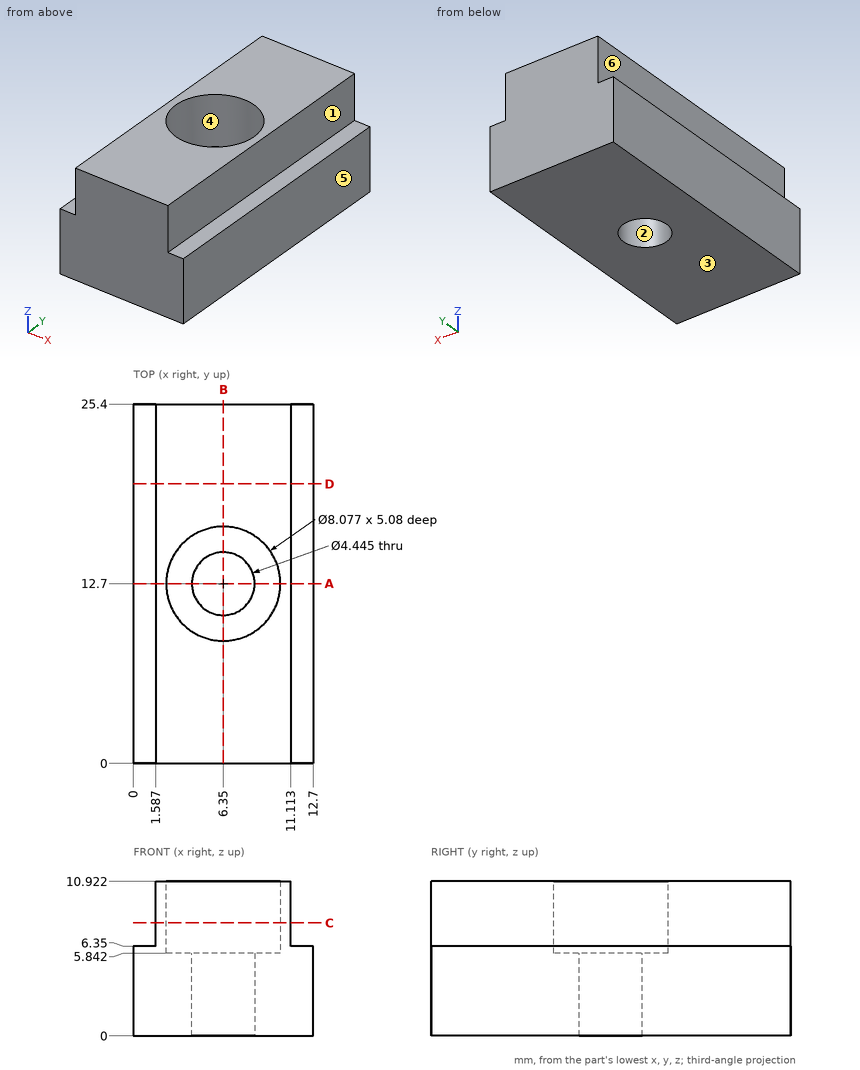
Here's the drawing with two shaded views (mm, measured from the low corner). I have some questions. A direction names the side the tool comes from. Give positions to 0.01 mm unless a question says otherwise; leave off trailing zeros. Order: outer loops, then holes, each group sorted by start corner. A loop starts at its lowest first (then second) coordinate and runs counter-clockwise, first axis right, second up.
Q1. I'm going to push flat-ended pins straight in: P1, Ø2.5, axis at x = 6.35, y = 12.7, coming from the -Z side; P2, Ø5, axis at x = 6.35, y = 12.7, coming from the +Z side; P3, Ø1.4, axis at y = 13.5, z = 9, coming from the -X side. Where does each tip first touch, or does it pass through?
Q2. If I drill on line 1 along Y through (x, z) = (6.35, 9.45); line 2 along Y through (x, z) = (6.35, 2.4); line 3 along Z through (x, y) = (5.5, 10.5), over which ranges is the centre line in solid material (lowest first)?
Q3. Suppose I cut it at A-A, the plane y = 12.7. Write out the boundary of the cut face in (x, z).
Q4. Suppose I cut it at C-C, the plane z = 8. Write out the boundary of the cut face in (x, y), and give its area (3 significant figures).
Q5. We'd pull the mould along X, two halves only. Please class the marked faces 3, 4, 5 and 6: +X half, -X half, draft (parallel to the pull), parting line (faces both ways), or undercut.
Q6. For the marked faces 1 and 2, which set-ups out of +Z, -Z, +X, -X, +Y, -Y let a thin tool reach every point of the face, with its end or its side?
Q7. Suppose I cut it at D-D, the plane y = 19.75. Write out the boundary of the cut face in (x, z).
Q8. Suppose I cut it at B-B, the plane x = 6.35. Write out the boundary of the cut face in (y, z).
Solution:
1. P1: passes through
1. P2: stops at z = 5.84
1. P3: stops at x = 1.59
2. line 1: y = 0 to 8.66, 16.74 to 25.4
2. line 2: y = 0 to 10.48, 14.92 to 25.4
2. line 3: z = 0 to 5.84
3. outline: (0, 0) - (4.13, 0) - (4.13, 5.84) - (2.31, 5.84) - (2.31, 10.92) - (1.59, 10.92) - (1.59, 6.35) - (0, 6.35) - close; (8.57, 0) - (12.7, 0) - (12.7, 6.35) - (11.11, 6.35) - (11.11, 10.92) - (10.39, 10.92) - (10.39, 5.84) - (8.57, 5.84) - close
4. outline: (1.59, 0) - (11.11, 0) - (11.11, 25.4) - (1.59, 25.4) - close; hole circle Ø8.08 at (6.35, 12.7)
4. area: 191 mm2
5. face 3: draft
5. face 4: undercut
5. face 5: +X half
5. face 6: -X half
6. face 1: +Z, +X, +Y, -Y
6. face 2: +Z, -Z
7. outline: (0, 0) - (12.7, 0) - (12.7, 6.35) - (11.11, 6.35) - (11.11, 10.92) - (1.59, 10.92) - (1.59, 6.35) - (0, 6.35) - close
8. outline: (0, 0) - (10.48, 0) - (10.48, 5.84) - (8.66, 5.84) - (8.66, 10.92) - (0, 10.92) - close; (14.92, 0) - (25.4, 0) - (25.4, 10.92) - (16.74, 10.92) - (16.74, 5.84) - (14.92, 5.84) - close
